Read the model definition and answer for the solid it produces. Units are mm, in the model's axes. Face numbers are marked on the shaded views. A direction names the side the tool comes from. Round coordinates to 2 decimals unless told otherwise and drop trailing zeros. Write each loop counter-clockwise with the first axis right and the second up, starting at its lowest first coordinate (ties: lowest second). Pieces come first, ordered by that corner, then holes. Notation, with made-up numbers: (-21.5, 86.25) - (-17.5, 86.25) arc R21 ccw to (-17.5, 94.25) - close; hole circle Ø4 at (-27.75, 77.5). An arc over 180 degrees is marked (long way). One line per item, written item: value. Start each with the question number.
(1) Flat-ended cylindrical pins translate along their axes: pin 1 Ø5 at (x, y) = (6, 3.5) entering from -Z; pin 2 Ø4 at (y, z) = (0, 30) entering from +X. Find the tip coordinate at first contact, or state that the pin passes through.
(2) Find the intervals of material crossed by L1, parallel to Y at x = 9.4, z = -10; L2, parallel to X at y = -8.75, z = 0, in increasing order.
(3) For the marked faces 4 and 5, determine the directions among +Z, -Z, +X, -X, +Y, -Y from which every point of the face is accessible in a straight line to the end or side of a thin tool.
(4) The mould has two halves that part along X. Classify the marked faces 1, 2 and 3: +X half, -X half, draft (parallel to the pull), parting line (faces both ways), or undercut.
(5) A cutting plane is placed at C-C, the plane z = -14. Determine the outline of the cut face in (x, y), plus the area to 3 significant figures.
(6) A cutting plane is placed at A-A, the plane x = 4.25. Determine the outline of the cut face in (y, z), plus the area to 3 significant figures.
from build123d import *

# Parameters (mm, degrees)
SKETCH_1_W          = 20
SKETCH_1_H          = 20
SKETCH_1_W_2        = 18
SKETCH_1_H_2        = 18
EXTRUDE_1_DEPTH     = 40
SKETCH_2_R          = 1.5
CUT_EXTRUDE_1_DEPTH = 200
SKETCH_3_R          = 1.5
CUT_EXTRUDE_2_DEPTH = 40


with BuildPart() as part:
    # 草图1 → 凸台-拉伸1 (new, symmetric)
    with BuildSketch(Plane.XY):
        Rectangle(SKETCH_1_W, SKETCH_1_H)
        Rectangle(SKETCH_1_W_2, SKETCH_1_H_2, mode=Mode.SUBTRACT)
    extrude(amount=EXTRUDE_1_DEPTH, both=True)

    # 草图2 → 切除-拉伸1 (cut)
    with BuildSketch(Plane(origin=(0, 10, 0), x_dir=(1, 0, 0), z_dir=(0, 1, 0))):
        with Locations(Location((0, -20, 0), (0, 0, 270))):
            Circle(SKETCH_2_R)
        with Locations(Location((0, 0, 0), (0, 0, 270))):
            Circle(SKETCH_2_R)
    extrude(amount=-CUT_EXTRUDE_1_DEPTH, mode=Mode.SUBTRACT)

    # 草图3 → 切除-拉伸2 (cut)
    with BuildSketch(Plane.ZY.offset(10)):
        with Locations((10, 0)):
            Circle(SKETCH_3_R)
        with Locations((-10, 0)):
            Circle(SKETCH_3_R)
        with Locations((30, 0)):
            Circle(SKETCH_3_R)
        with Locations((-30, 0)):
            Circle(SKETCH_3_R)
    extrude(amount=-CUT_EXTRUDE_2_DEPTH, mode=Mode.SUBTRACT)


solid = part.part
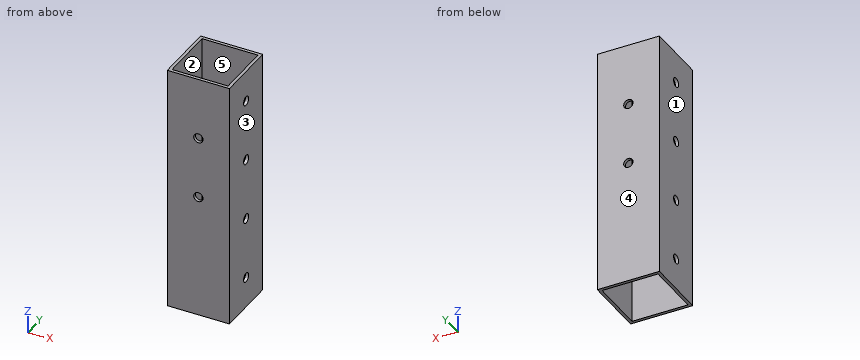
Here are the results:
1. pin 1: through
1. pin 2: x = 10
2. L1: -10 to -1.5, 1.5 to 10
2. L2: -10 to -9, 9 to 10
3. face 4: +Z, -Z, +X, -X, +Y
3. face 5: +Z, -Z
4. face 1: -X half
4. face 2: undercut
4. face 3: +X half
5. outline: (-10, -10) - (10, -10) - (10, 10) - (-10, 10) - close; hole (-9, -9) - (9, -9) - (9, 9) - (-9, 9) - close
5. area: 76.0 mm²
6. outline: (-10, -40) - (-9, -40) - (-9, 40) - (-10, 40) - close; (9, -40) - (10, -40) - (10, 40) - (9, 40) - close
6. area: 160 mm²
